Design review of the part built by this model. Coordinates are the model's own, in mm. A direction names the side the tool comes from. Give positions to 0.01 mm unless a question says otherwise; leave off trailing zeros. Write each loop counter-clockwise with the first axis right and the second up, starting at its lowest first coordinate (ties: lowest second). Pieces come first, ordered by that corner, then holes. Notation, with made-up numbers: (61.5, -35) -> (96.5, -35) arc R9 ccw to (96.5, -31) -> close; hole circle Ø3 at (47, 85.5). An arc over 180 degrees is marked (long way). Use CSV: the item, a comma, the result in double quotes.
```python
from build123d import *

# Parameters (mm, degrees)
F0_W     = 320
F0_H     = 320
F0_W_2   = 300
F0_H_2   = 300
F1_DEPTH = 800
F2_W     = 400
F2_H     = 400
F2_W_2   = 300
F2_H_2   = 300
F3_DEPTH = 10


with BuildPart() as f1:
    # F0 (on Top) → F1 (new body)
    with BuildSketch(Plane.XY):
        Rectangle(F0_W, F0_H)
        Rectangle(F0_W_2, F0_H_2, mode=Mode.SUBTRACT)
    extrude(amount=F1_DEPTH)

    # F2 (on face) + F0 (on Top) → F3 (join)
    with BuildSketch(Plane.XY):
        Rectangle(F2_W, F2_H)
        Rectangle(F2_W_2, F2_H_2, mode=Mode.SUBTRACT)
    with BuildSketch(Plane.XY):
        Rectangle(F0_W_2, F0_H_2)
    extrude(amount=-F3_DEPTH)


solid = f1.part
```
(1) For line 1 along Y through (x, z) = (-22, 753.5); line 2 along Z through (x, y) = (-80.5, 44), list the stretches that pass through material, from the lowest coordinate up. Write a range as [from, to].
Established:
line 1,"y = [-160, -150], [150, 160]"
line 2,"z = [-10, 0]"
(2) Take a section at D-D (y = 176). Write out the cut boundary in (x, z), then the cut area to 3 significant figures.
Established:
outline,"(-200, -10) -> (200, -10) -> (200, 0) -> (-200, 0) -> close"
area,"4,000 mm2"
(3) Take a section at A-A (z = 462). Write out the cut boundary in (x, y), then the cut area to 3 significant figures.
Established:
outline,"(-160, -160) -> (160, -160) -> (160, 160) -> (-160, 160) -> close; hole (-150, -150) -> (150, -150) -> (150, 150) -> (-150, 150) -> close"
area,"12,400 mm2"
(4) Tool access review of faces 5 (the face through (-160, -2, 394)), 6 (the face through (160, -2, 394)), 7 (the face through (-2, 2, 0)), 8 (the face through (-13, -153, 800)): name each direction out of +Z, -Z, +X, -X, +Y, -Y from which nothing blocks a thin tool from reaching the whole face with its end or side.
Established:
face 5,"+Z, -X, +Y, -Y"
face 6,"+Z, +X, +Y, -Y"
face 7,"+Z"
face 8,"+Z, +X, -X, +Y, -Y"
(5) Take a section at B-B (x = 25.5). Write out the cut boundary in (y, z).
Established:
outline,"(-200, -10) -> (200, -10) -> (200, 0) -> (160, 0) -> (160, 800) -> (150, 800) -> (150, 0) -> (-150, 0) -> (-150, 800) -> (-160, 800) -> (-160, 0) -> (-200, 0) -> close"
(6) Mouldability with a two-part tool opening along Y and no side actions: class faces 1 (the face through (-2, -160, 394)), 2 (the face through (-3, 3, -10)), 3 (the face through (-2, 160, 394)), 4 (the face through (150, -2, 394)) as +Y half, -Y half, draft (parallel to the pull), parting line (faces both ways), or undercut.
Established:
face 1,"-Y half"
face 2,"draft"
face 3,"+Y half"
face 4,"undercut"
(7) Clearance check with flat-ended pins moving along their axes: pin 1 (10 mm diameter, centred on x = -142, z = 604.5, fed in from -Y); pin 2 (3 mm diameter, centred on y = 124.5, z = 406, fed in from -X); pin 3 (1.5 mm diameter, centred on y = -6.5, z = 97, fed in from +X). State where each tip first meets the part, or that it passes through.
Established:
pin 1,"stops at y = -160"
pin 2,"stops at x = -160"
pin 3,"stops at x = 160"
